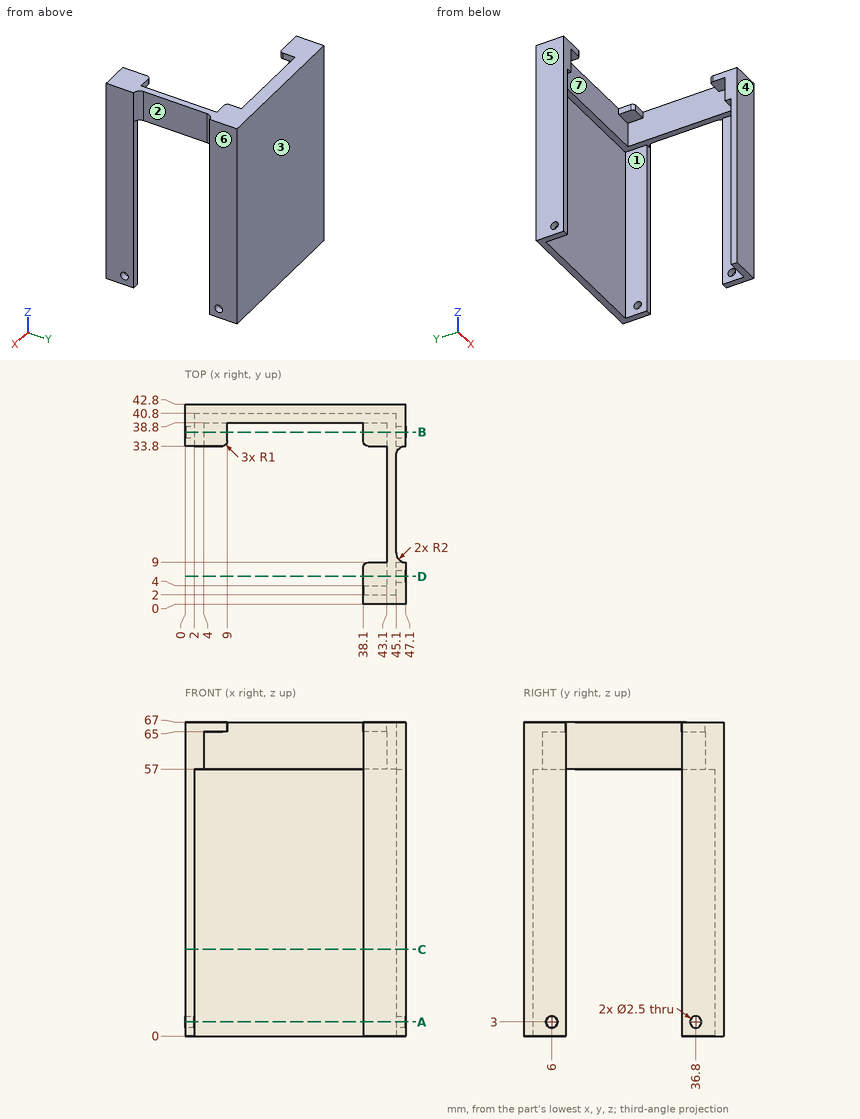
Input: dimensioned drawing with shaded views. Units: mm. Origin: part minimum x, y, z. A direction names the side the tool comes from. Round coordinates to 2 decimals unless told otherwise and drop trailing zeros. Order: outer loops, then holes, each group sorted by start corner. A loop starts at its lowest first (then second) coordinate and runs counter-clockwise, first axis right, second up.
Q1. Mould query, pull axis X, two halves, no side actions, for the marked faces 4, 5, 6 and 7. Classes: released by +X, released by -X, zero draft, split by the parting line, or undercut.
Result sheet:
face 4: zero draft
face 5: released by -X
face 6: released by +X
face 7: undercut
Q2. Section A-A, the plane z = 3. Output: boundary loops of the cut face in (x, y), and give its area (3 significant figures).
Result sheet:
outline: (0, 33.8) - (2, 33.8) - (2, 35.55) - (0, 35.55) - close; (0, 38.05) - (2, 38.05) - (2, 40.8) - (45.1, 40.8) - (45.1, 38.05) - (47.1, 38.05) - (47.1, 42.8) - (0, 42.8) - close; (38.1, 0) - (47.1, 0) - (47.1, 4.75) - (45.1, 4.75) - (45.1, 2) - (38.1, 2) - close; (45.1, 7.25) - (47.1, 7.25) - (47.1, 9) - (45.1, 9) - close; (45.1, 33.8) - (47.1, 33.8) - (47.1, 35.55) - (45.1, 35.55) - close
area: 139 mm2
Q3. Section D-D, the plane y = 6. Output: boundary loops of the cut face in (x, z), and give its area (3 significant figures).
Result sheet:
outline: (38.1, 65) - (43.1, 65) - (43.1, 57) - (45.1, 57) - (45.1, 4.25) - (47.1, 4.25) - (47.1, 67) - (38.1, 67) - close; (45.1, 0) - (47.1, 0) - (47.1, 1.75) - (45.1, 1.75) - close
area: 159 mm2
Q4. Pin query (flat end, axial travel): pin 1 (2.5 mm diameter, centred on x = 4, z = 23, fed in from -Y); pin 2 (4 mm diameter, centred on x = 39.5, y = 7, fed in from -Z); pin 3 (5.5 mm diameter, centred on y = 5, z = 16, fed in from -X). Return the tip coordinate at first contact, or that it passes through.
Result sheet:
pin 1: stops at y = 40.8
pin 2: stops at z = 65
pin 3: stops at x = 45.1
Q5. Section B-B, the plane y = 36.8. Output: boundary loops of the cut face in (x, z).
Result sheet:
outline: (0, 0) - (2, 0) - (2, 1.75) - (0, 1.75) - close; (0, 4.25) - (2, 4.25) - (2, 57) - (4, 57) - (4, 65) - (9, 65) - (9, 67) - (0, 67) - close; (38.1, 65) - (43.1, 65) - (43.1, 57) - (45.1, 57) - (45.1, 4.25) - (47.1, 4.25) - (47.1, 67) - (38.1, 67) - close; (45.1, 0) - (47.1, 0) - (47.1, 1.75) - (45.1, 1.75) - close
Q6. Section C-C, the plane z = 18.5. Output: boundary loops of the cut face in (x, y).
Result sheet:
outline: (0, 33.8) - (2, 33.8) - (2, 40.8) - (45.1, 40.8) - (45.1, 33.8) - (47.1, 33.8) - (47.1, 42.8) - (0, 42.8) - close; (38.1, 0) - (47.1, 0) - (47.1, 9) - (45.1, 9) - (45.1, 2) - (38.1, 2) - close
Q7. Material intervals for probe 1 along Y at (x, z) = (45.5, 3); probe 2 along Y at (x, z) = (40, 22); probe 3 along Z at (x, y) = (46.25, 6), sorted ascending.
Result sheet:
probe 1: y = 0 to 4.75, 7.25 to 9, 33.8 to 35.55, 38.05 to 42.8
probe 2: y = 0 to 2, 40.8 to 42.8
probe 3: z = 0 to 1.75, 4.25 to 67
Q8. Access query for the marked faces 1, 2 and 3. Directions: +Z, -Z, +X, -X, +Y, -Y. A direction counts if a zero-diameter tool reaches every point of the face in a straight line with its end or side. Return the directions, or none.
Result sheet:
face 1: -Z
face 2: +Z, -Z, +X
face 3: +Z, -Z, +X, -X, +Y
